from build123d import *

# Parameters (mm, degrees)
SKETCH1_W                                    = 50
SKETCH1_H                                    = 112
SKETCH1_W_2                                  = 24
SKETCH1_H_2                                  = 18
BOSS_EXTRUDE1_DEPTH                          = 10
SKETCH8_W                                    = 36
SKETCH8_H                                    = 50
SKETCH8_H_2                                  = 18
CUT_EXTRUDE1_DEPTH                           = 116.191145493
CBORE_FOR_M3_HEXAGON_SOCKET_HEAD_CAP_2_COUNT = 2
CBORE_FOR_M3_HEXAGON_SOCKET_HEAD_CAP_2_PITCH = 12
CBORE_FOR_M3_HEXAGON_SOCKET_HEAD_CAP_3_COUNT = 2
CBORE_FOR_M3_HEXAGON_SOCKET_HEAD_CAP_3_PITCH = 29
CBORE_FOR_M3_HEXAGON_SOCKET_HEAD_CAP_4_COUNT = 2
CBORE_FOR_M3_HEXAGON_SOCKET_HEAD_CAP_4_PITCH = 31.384709653
CHAMFER1_SIZE                                = 1
FILLET1_R                                    = 2
M3_TAPPED_HOLE1_D                            = 2.5
M3_TAPPED_HOLE1_DEPTH                        = 9.5
M3_TAPPED_HOLE1_CSINK_D                      = 3.05
M3_TAPPED_HOLE1_CSINK_ANGLE                  = 90
M3_TAPPED_HOLE1_TIP                          = 0.751075774


with BuildPart() as part:
    # Sketch1 → Boss-Extrude1 (new body)
    with BuildSketch(Plane.XY):
        with Locations((0, -56)):
            Rectangle(SKETCH1_W, SKETCH1_H)
        with Locations((0, -17)):
            Rectangle(SKETCH1_W_2, SKETCH1_H_2, mode=Mode.SUBTRACT)
    extrude(amount=BOSS_EXTRUDE1_DEPTH)

    # Sketch8 → Cut-Extrude1 (cut, through all)
    with BuildSketch(Plane.XY.offset(10)):
        with Locations((0, -56)):
            Rectangle(SKETCH8_W, SKETCH8_H)
        with Locations((0, -95)):
            Rectangle(SKETCH8_W, SKETCH8_H_2)
    extrude(amount=-CUT_EXTRUDE1_DEPTH, mode=Mode.SUBTRACT)

    # Sketch7 → CBORE for M3 Hexagon socket head cap screws3 (revolve, cut)
    with BuildSketch(Plane(origin=(-14.5, -4, 10), x_dir=(0, -1, 0), z_dir=(1, 0, 0))):
        Polygon((0, 0), (0, 10), (1.6, 10), (1.6, 3.4), (3, 3.4), (3, 0.025), (3.025, 0), align=None)
    cbore_for_m3_hexagon_socket_head_cap_scr = revolve(axis=Axis((-14.5, -4, 16.35), (0, 0, -1)), mode=Mode.SUBTRACT)

    # CBORE for M3 Hexagon socket head cap 2: CBORE for M3 Hexagon socket head cap screws3 ×2
    with Locations(*[(0, -i * CBORE_FOR_M3_HEXAGON_SOCKET_HEAD_CAP_2_PITCH, 0) for i in range(1, CBORE_FOR_M3_HEXAGON_SOCKET_HEAD_CAP_2_COUNT)]):
        add(cbore_for_m3_hexagon_socket_head_cap_scr, mode=Mode.SUBTRACT)

    # CBORE for M3 Hexagon socket head cap 3: CBORE for M3 Hexagon socket head cap screws3 ×2
    with Locations(*[(i * CBORE_FOR_M3_HEXAGON_SOCKET_HEAD_CAP_3_PITCH, 0, 0) for i in range(1, CBORE_FOR_M3_HEXAGON_SOCKET_HEAD_CAP_3_COUNT)]):
        add(cbore_for_m3_hexagon_socket_head_cap_scr, mode=Mode.SUBTRACT)

    # CBORE for M3 Hexagon socket head cap 4: CBORE for M3 Hexagon socket head cap screws3 ×2
    with Locations(*[Vector(0.9240168324218909, -0.38235179272629954, 0) * (i * CBORE_FOR_M3_HEXAGON_SOCKET_HEAD_CAP_4_PITCH) for i in range(1, CBORE_FOR_M3_HEXAGON_SOCKET_HEAD_CAP_4_COUNT)]):
        add(cbore_for_m3_hexagon_socket_head_cap_scr, mode=Mode.SUBTRACT)

    # Chamfer1
    chamfer1_edges = [part.edges().sort_by_distance(p)[0] for p in [
        (-25, 0, 5),
        (25, 0, 5),
    ]]
    chamfer(chamfer1_edges, length=CHAMFER1_SIZE)

    # Fillet1
    fillet1_edges = [part.edges().sort_by_distance(p)[0] for p in [
        (-12, -8, 5),
        (-12, -26, 5),
        (12, -26, 5),
        (12, -8, 5),
        (-12, -14.341687605, 8.2875),
        (-12, -17.658312395, 8.2875),
        (12, -17.658312395, 8.2875),
        (12, -14.341687605, 8.2875),
        (18, -86, 5),
        (18, -104, 5),
        (-18, -104, 5),
        (-18, -86, 5),
        (18, -31, 5),
        (18, -81, 5),
        (-18, -81, 5),
        (-18, -31, 5),
    ]]
    fillet(fillet1_edges, radius=FILLET1_R)

    # M3 Tapped Hole1
    with Locations(Plane(origin=(-21.75, -112, 5), x_dir=(0, 0, -1), z_dir=(0, -1, 0))):
        with Locations((0, 0), (0, 43.5)):
            CounterSinkHole(M3_TAPPED_HOLE1_D / 2, M3_TAPPED_HOLE1_CSINK_D / 2, depth=M3_TAPPED_HOLE1_DEPTH, counter_sink_angle=M3_TAPPED_HOLE1_CSINK_ANGLE)
            with Locations((0, 0, -(M3_TAPPED_HOLE1_DEPTH + M3_TAPPED_HOLE1_TIP / 2))):  # 118° drill point
                Cone(0, M3_TAPPED_HOLE1_D / 2, M3_TAPPED_HOLE1_TIP, mode=Mode.SUBTRACT)


solid = part.part
Check sheet for the modelled part. Datum: model origin and axes. Units: mm. A direction names the side the tool comes from. Round coordinates to 2 decimals unless told otherwise and drop trailing zeros. Loops run counter-clockwise (first coordinate to the right, second up) from the corner with the lowest first, then second, coordinate; pieces in that order, holes last. Notation, with made-up numbers: (66.25, -26.75) -> (111.25, -26.75) arc R13 ccw to (111.25, -1.75) -> close; hole circle Ø9 at (65, 34.25). An arc over 180 degrees is marked (long way). Put each result on its own line as item: value. Start each with the question number.
1. Scan lines: probe 1 along Y at (x, z) = (-2, 5.5); probe 2 along X at (y, z) = (-105.75, 5); probe 3 along X at (y, z) = (-16, 5.5). Record each from-to range of solid material in increasing order.
2. Section check B-B (y = -96.5). Enter the section's corners in (x, z).
3. Access from +Z, -Z, +X, -X, +Y, -Y to the whole of each face (thin tool, end or side, straight path). Record for faces 1 (the face through (-23, -107, 5)), 2 (the face through (13, -15, 6.6)), 3 (the face through (17.4, -80.43, 4.93)).
4. Gauge pin test, flat end, axial feed: pin 1 (1.6 mm diameter, centred on x = -15, y = -18, fed in from +Z). Record the tip position at first contact, or that the pin passes through.
5. Draft check along Y on faces 4 (the face through (12.64, -12.49, 8.32)), 5 (the face through (20.53, -107.05, 4.73)), 6 (the face through (0, 0, 5)). Enter one of: +Y half, -Y half, draft (parallel to the pull), parting line (faces both ways), or undercut.
6. Section check A-A (x = -7.5). Enter the section's corners in (y, z).
7. Section check D-D (z = 8.25). Give the number of separate pieces and of enclosed holes in the cut face, plus the area to 3 significant figures.
8. Section check C-C (y = -4). Enter the section's corners in (x, z) (3 decimals), plus the area to 3 significant figures.
Findings:
1. probe 1: y = -112 to -104, -86 to -81, -31 to -26, -8 to 0
1. probe 2: x = -25 to -23, -20.5 to 20.5, 23 to 25
1. probe 3: x = -25 to -16.1, -12.9 to -12, 12 to 12.9, 16.1 to 25
2. outline: (-25, 0) -> (-18, 0) -> (-18, 10) -> (-25, 10) -> close; (18, 0) -> (25, 0) -> (25, 10) -> (18, 10) -> close
3. face 1: -Y
3. face 2: +Z
3. face 3: +Z, -Z
4. pin 1: stops at z = 6.6
5. face 4: undercut
5. face 5: draft
5. face 6: +Y half
6. outline: (-112, 0) -> (-104, 0) -> (-104, 10) -> (-112, 10) -> close; (-86, 0) -> (-81, 0) -> (-81, 10) -> (-86, 10) -> close; (-31, 0) -> (-26, 0) -> (-26, 10) -> (-31, 10) -> close; (-8, 0) -> (0, 0) -> (0, 10) -> (-8, 10) -> close
7. separate pieces: 1
7. enclosed holes: 5
7. area: 2,610 mm^2
8. outline: (-25, 0) -> (-16.1, 0) -> (-16.1, 6.6) -> (-17.5, 6.6) -> (-17.5, 9.975) -> (-17.525, 10) -> (-25, 10) -> close; (-12.9, 0) -> (12.9, 0) -> (12.9, 6.6) -> (11.5, 6.6) -> (11.5, 9.975) -> (11.475, 10) -> (-11.475, 10) -> (-11.5, 9.975) -> (-11.5, 6.6) -> (-12.9, 6.6) -> close; (16.1, 0) -> (25, 0) -> (25, 10) -> (17.525, 10) -> (17.5, 9.975) -> (17.5, 6.6) -> (16.1, 6.6) -> close
8. area: 417 mm^2
